from build123d import *

# Parameters (mm, degrees)
SKETCH1_R           = 8
BOSS_EXTRUDE1_DEPTH = 35
CUT_EXTRUDE1_DEPTH  = 14
SKETCH1_4_R         = 5
CUT_EXTRUDE2_DEPTH  = 15.5
CUT_EXTRUDE3_REACH  = 26
SKETCH5_R           = 7.25


with BuildPart() as part:
    # Sketch1 → Boss-Extrude1 (new body)
    with BuildSketch(Plane(origin=(0, 0, 0), x_dir=(1, 0, 0), z_dir=(0, 1, 0))):
        Circle(SKETCH1_R)
    extrude(amount=BOSS_EXTRUDE1_DEPTH)

    # Sketch1_3 → Cut-Extrude1 (cut)
    with BuildSketch(Plane(origin=(0, 0, 0), x_dir=(1, 0, 0), z_dir=(0, 1, 0))):
        with BuildLine():
            Line((6.92820323, 4), (6.92820323, -4))
            ThreePointArc((6.92820323, -4), (7.72740661, -2.070552361), (8, 0))
            ThreePointArc((8, 0), (7.72740661, 2.070552361), (6.92820323, 4))
        make_face()
        with BuildLine():
            ThreePointArc((-6.92820323, 4), (-8, 0), (-6.92820323, -4))
            Line((-6.92820323, -4), (-6.92820323, 4))
        make_face()
    extrude(amount=CUT_EXTRUDE1_DEPTH, mode=Mode.SUBTRACT)

    # Sketch1_4 → Cut-Extrude2 (cut)
    with BuildSketch(Plane(origin=(0, 0, 0), x_dir=(1, 0, 0), z_dir=(0, 1, 0))):
        Circle(SKETCH1_4_R)
    extrude(amount=CUT_EXTRUDE2_DEPTH, mode=Mode.SUBTRACT)

    # Sketch2 one side → Revolve13 (revolve)
    with BuildSketch(Plane(origin=(0, 0, 0), x_dir=(0, 0, -1), z_dir=(1, 0, 0))):
        with BuildLine():
            Line((0, 23), (0, 47))
            ThreePointArc((0, 47), (-12, 35), (0, 23))
        make_face()
    revolve(axis=Axis((0, 35, 0), (0, 1, 0)))

    # Sketch4 one side → Cut-Revolve2 (revolve, cut)
    with BuildSketch(Plane(origin=(0, 0, 0), x_dir=(0, 0, -1), z_dir=(1, 0, 0))):
        with BuildLine():
            ThreePointArc((6.84, 35), (4.496854249, 40.656854249), (-1.16, 43))
            Line((-1.16, 43), (-1.16, 27))
            ThreePointArc((-1.16, 27), (4.496854249, 29.343145751), (6.84, 35))
        make_face()
    revolve(axis=Axis((0, 27, 1.16), (0, -1, 0)), mode=Mode.SUBTRACT)

    # Sketch5 → Cut-Extrude3 (cut, up to next)
    with BuildSketch(Plane.XY.offset(12), mode=Mode.PRIVATE) as cut_extrude3_sk1:
        with Locations((0, 35)):
            Circle(SKETCH5_R)
    cut_extrude3_tool1 = extrude(cut_extrude3_sk1.sketch, amount=-CUT_EXTRUDE3_REACH, mode=Mode.PRIVATE) & part.part
    add(cut_extrude3_tool1.solids().sort_by_distance((0, 35, 12))[0], mode=Mode.SUBTRACT)


solid = part.part
Check sheet for the modelled part. Datum: model origin and axes. Units: mm. A direction names the side the tool comes from. Coordinates: 2 decimals unless noted, no trailing zeros. Loops run counter-clockwise (first coordinate to the right, second up) from the corner with the lowest first, then second, coordinate; pieces in that order, holes last. Notation, with made-up numbers: (-32, -28.5) -> (18, -28.5) arc R19 ccw to (18, -7.5) -> close; hole circle Ø10 at (74.25, 65). An arc over 180 degrees is marked (long way). Write item = value, one per line. Start each with the question number.
1. Depth check by flat-ended pin: P1, Ø12, axis at x = 8, y = 31, coming from the -Z side; P2, Ø2, axis at x = 7, y = 8.5, coming from the +Z side; P3, Ø10, axis at y = 25.5, z = 4, coming from the -X side. Enter the tip coordinate at first touch or a pass-through.
2. Material ranges on line 1 (X direction, y = 5.5, z = 0); line 2 (Z direction, x = 0, y = 11.75); line 3 (Z direction, x = -6.25, y = 18.5), recorded low to high.
3. Section check B-B on x = 0. Record the cut outline in (y, z), then the cut area to 3 significant figures.
4. Section check C-C on z = 0. Record the cut outline in (x, y).
5. Section check D-D on y = 19. Record the cut outline in (x, z).
6. Tool access check on faces 5 (the cylindrical face through (-1.57, 27.92, 7.09)), 6 (the flat face through (-7.4, 14, -0.1)), 7 (the flat face through (6.928, 7, 0)). Record the directions out of +Z, -Z, +X, -X, +Y, -Y that give a thin tool (end or side, any length) a straight path to the whole face; none if there is none.
7. Section check A-A on y = 6. Record the cut outline in (x, z), then the cut area to 3 significant figures.
8. Draft check along Z on faces 1 (the cylindrical face through (-1.08, 7.64, 4.88)), 2 (the cylindrical face through (-8, 16, 0)), 3 (the flat face through (0, 15.5, 0)), 4 (the flat face through (-6.928, 7, 0)). Enter one of: released by +Z, released by -Z, zero draft, split by the parting line, or undercut.
Responses:
q1.P1 = -11.63
q1.P2 = 5.29
q1.P3 = -10.76
q2.line_1 = -6.93 to -5, 5 to 6.93
q2.line_2 = -8 to -5, 5 to 8
q2.line_3 = -4.99 to 4.99
q3.outline = (0, -8) -> (26.06, -8) arc R12 ccw (long way) to (42.25, 9.56) -> (42.25, 4.54) arc R8 cw (long way) to (27.75, 4.54) -> (27.75, 9.56) arc R12 ccw to (26.06, 8) -> (0, 8) -> (0, 5) -> (15.5, 5) -> (15.5, -5) -> (0, -5) -> close
q3.area = 431 mm2
q4.outline = (-8, 14) -> (-6.93, 14) -> (-6.93, 0) -> (-5, 0) -> (-5, 15.5) -> (5, 15.5) -> (5, 0) -> (6.93, 0) -> (6.93, 14) -> (8, 14) -> (8, 26.06) arc R12 ccw (long way) to (-8, 26.06) -> close; hole circle Ø15.83 at (0, 35)
q5.outline = circle Ø16 at (0, 0)
q6.face_5 = +Z
q6.face_6 = +Z, -Z, -X, -Y
q6.face_7 = +Z, -Z, +X, -Y
q7.outline = (-6.93, -4) arc R8 ccw to (6.93, -4) -> (6.93, 4) arc R8 ccw to (-6.93, 4) -> close; hole circle Ø10 at (0, 0)
q7.area = 111 mm2
q8.face_1 = undercut
q8.face_2 = split by the parting line
q8.face_3 = undercut
q8.face_4 = zero draft
